Check sheet for the modelled part. Datum: model origin and axes. Units: mm. A direction names the side the tool comes from. Coordinates: 2 decimals unless noted, no trailing zeros. Order: outer loops, then holes, each group sorted by start corner. A loop starts at its lowest first (then second) coordinate and runs counter-clockwise, first axis right, second up. Notation, with made-up numbers: M -24,85.5 L 8,85.5 A23 cw 8,120.5 Z; hole C 11,-19 d3. An arc over 180 degrees is marked long. Answer in a Markdown table with one row per item. Add a question column.
Autodesk Inventor part; units mm, degrees
ref_plane "YZ Plane" through (0, 0, 0) normal (1, 0, 0) x (0, 1, 0)
ref_plane "XZ Plane" through (0, 0, 0) normal (0, 1, 0) x (-1, 0, 0)
ref_plane "XY Plane" through (0, 0, 0) normal (0, 0, 1) x (1, 0, 0)
sketch "Sketch1" plane through (0, 0, 0) normal (0, 0, 1) x (1, 0, 0)
  circle A0 centre (0, 0) radius 3.75
  line L0 (-10, 10) -> (10, 10)
  line L1 (10, 10) -> (10, -10)
  line L2 (10, -10) -> (-10, -10)
  line L3 (-10, -10) -> (-10, 10)
  line L4 (-10, 10) -> (10, -10) construction
  line L5 (10, 10) -> (-10, -10) construction
  dimension "d0" = 7.5
  dimension "d1" = 20
  dimension "d2" = 20
extrude "Extrusion1" add sketch "Sketch1" along normal blind 4
sketch "Sketch2" plane through (-10, 10, 0) normal (0, 1, 0) x (1, 0, 0)
  line L0 (20, -4) -> (0, -4)
  line L1 (0, -4) -> (20, -4)
  line L2 (20, -4) -> (20, 20)
  line L3 (20, 20) -> (0, 20)
  line L4 (0, 20) -> (0, -4)
  point P0 (10, 0)
  dimension "d5" = 24
extrude "Extrusion2" add sketch "Sketch2" along normal blind 4
sketch "Sketch3" plane through (10, -10, 4) normal (1, 0, 0) x (0, 0, -1)
  line L0 (4, 0) -> (0, 0)
  line L1 (4, 20) -> (24, 20)
  line L2 (4, 0) -> (24, 20)
  line L3 (24, 20) -> (24, 24)
  line L4 (24, 20) -> (24, 24)
  line L5 (24, 24) -> (0, 24)
  line L6 (24, 24) -> (0, 24)
  line L7 (0, 0) -> (0, 24)
  line L8 (0, 24) -> (0, 0)
  line L9 (0, 0) -> (4, 0)
  point P0 (4, 10)
extrude "Extrusion3" add sketch "Sketch3" along normal blind 4
ref_plane "Work Plane1" through (0, -10, 4) normal (1, 0, 0) x (0, 0, -1)
mirror "Mirror1" about plane through (0, -10, 4) normal (1, 0, 0) of "Extrusion3"
sketch "Sketch4" plane through (14, 10, -20) normal (0, 0, -1) x (-1, 0, 0)
  line L0 (3.5, 0) -> (24.5, 0)
  line L1 (24.5, 0) -> (24.5, -20)
  line L2 (24.5, -20) -> (3.5, -20)
  line L3 (3.5, -20) -> (3.5, 0)
  line L4 (3.5, 0) -> (24.5, -20) construction
  line L5 (24.5, 0) -> (3.5, -20) construction
  point P0 (14, -10)
  dimension "d11" = 21
  dimension "d12" = 20
extrude "Extrusion4" cut sketch "Sketch4" against normal blind 20
properties part number "Gabarito Furo BOX"
1. Section check A-A on y = 0. Enter the section's corners in (x, z).
2. Set-up check for faces 4 (the flat face through (0, 5, 4)), 5 (the flat face through (10.5, 4, -6)): record each of +Z, -Z, +X, -X, +Y, -Y from which the full face is reachable in a straight line by a thin tool's end or side.
3. Go/stop test with flat-tipped pins: pin 1 Ø2 at (x, y) = (6, 2) entering from -Z; pin 2 Ø10 at (x, z) = (1.5, -17.5) entering from -Y. Record where each tip stops, or that it passes through.
4. Release check for a two-part mould opening along X. For faces 1 (the flat face through (-14, 5, -6)), 2 (the flat face through (12, 0, -10)), 3 (the flat face through (0, 5, 0)) record: released by +X, released by -X, zero draft, split by the parting line, or undercut.
5. Section check B-B on x = 0. Enter the section's corners in (y, z).
6. Scan lines: line 1 (Y direction, x = 0, z = 2.15); line 2 (Y direction, x = -6, z = -18.25); line 3 (Z direction, x = -0.25, y = -4.5). Record each from-to range of solid material in increasing order.
Result sheet:
| question | item | result |
|---|---|---|
| 1 | outline | M -14,-10 L -10.5,-10 L -10.5,0 L -3.75,0 L -3.75,4 L -14,4 Z; M 3.75,0 L 10.5,0 L 10.5,-10 L 14,-10 L 14,4 L 3.75,4 Z |
| 2 | face 4 | +Z, +X, -X, +Y, -Y |
| 2 | face 5 | -Z, -Y |
| 3 | pin 1 | z = 0 |
| 3 | pin 2 | y = 10 |
| 4 | face 1 | released by -X |
| 4 | face 2 | zero draft |
| 4 | face 3 | undercut |
| 5 | outline | M -10,0 L -3.75,0 L -3.75,4 L -10,4 Z; M 3.75,0 L 10,0 L 10,-20 L 14,-20 L 14,4 L 3.75,4 Z |
| 6 | line 1 | -10 to -3.75, 3.75 to 14 |
| 6 | line 2 | 10 to 14 |
| 6 | line 3 | 0 to 4 |
